Verification items for the finished model (mm, model axes). Round coordinates to 2 decimals unless told otherwise and drop trailing zeros. Order: outer loops, then holes, each group sorted by start corner. A loop starts at its lowest first (then second) coordinate and runs counter-clockwise, first axis right, second up. Notation, with made-up numbers: M 80,7.5 L 134,7.5 A17 cw 134,18.5 Z; hole C -29,6.5 d9. An arc over 180 degrees is marked long. Use one line per item in the form item = value. Start each with the question number.
Item 1: Cross-section at B-B on x = 26. Enter the section's corners in (y, z), then the cut area to 3 significant figures.
Item 2: Cross-section at A-A on y = 30. Enter the section's corners in (x, z).
Item 3: Thickness scan on probe 1 along X at (y, z) = (19, 10); probe 2 along X at (y, z) = (72.5, 7.75); probe 3 along Y at (x, z) = (2.5, 8). Record the ranges inside material, lowest first. Write a range as [from, to].
Item 4: Go/stop test with flat-tipped pins: pin 1 Ø2 at (x, y) = (-2.5, -17.5) entering from -Z; pin 2 Ø3 at (x, y) = (25.58, 30) entering from +Z. Record where each tip stops, or that it passes through.
Item 5: Cross-section at C-C on x = -23.5. Enter the section's corners in (y, z).
Item 6: Release check for a two-part mould opening along Y. For faces 1 (the cylindrical face through (2.24, -66.03, 9.86)), 2 (the cylindrical face through (-24.96, 68.06, 9.86)), 3 (the flat face through (-1, 82, 10)), 4 (the flat face through (-37.5, -1, 10)) record: +Y half, -Y half, draft (parallel to the pull), parting line (faces both ways), or undercut.
from build123d import *

# Parameters (mm, degrees)
SKETCH1_W           = 75
SKETCH1_H           = 164
SKETCH1_R           = 1.4
SKETCH1_R_2         = 2.5
BOSS_EXTRUDE1_DEPTH = 20
SKETCH2_R           = 1.4
CUT_EXTRUDE1_DEPTH  = 165


with BuildPart() as part:
    # Sketch1 → Boss-Extrude1 (new body)
    with BuildSketch(Plane.XY):
        Rectangle(SKETCH1_W, SKETCH1_H)
        with Locations((-32.5324139, -64.662730375)):
            Circle(SKETCH1_R, mode=Mode.SUBTRACT)
        with Locations((32.436706201, -64.662730375)):
            Circle(SKETCH1_R, mode=Mode.SUBTRACT)
        with Locations((2.542, -64.662730375)):
            Circle(SKETCH1_R, mode=Mode.SUBTRACT)
        with Locations((25.583768895, 30)):
            Circle(SKETCH1_R_2, mode=Mode.SUBTRACT)
        with Locations((-24.416231105, 70.5)):
            Circle(SKETCH1_R_2, mode=Mode.SUBTRACT)
        with Locations((25.583768895, 70.5)):
            Circle(SKETCH1_R_2, mode=Mode.SUBTRACT)
        with Locations((-24.416231105, 30)):
            Circle(SKETCH1_R_2, mode=Mode.SUBTRACT)
    extrude(amount=BOSS_EXTRUDE1_DEPTH)

    # Sketch2 → Cut-Extrude1 (cut, through all)
    with BuildSketch(Plane(origin=(0, 82, 0), x_dir=(1, 0, 0), z_dir=(0, 1, 0))):
        with Locations((15.509889123, -9.995038215)):
            Circle(SKETCH2_R)
        with Locations((-15.490110877, -9.995038215)):
            Circle(SKETCH2_R)
    extrude(amount=-CUT_EXTRUDE1_DEPTH, mode=Mode.SUBTRACT)


solid = part.part
Output values:
q1.outline = M -82,0 L 27.53,0 L 27.53,20 L -82,20 Z; M 32.47,0 L 68.03,0 L 68.03,20 L 32.47,20 Z; M 72.97,0 L 82,0 L 82,20 L 72.97,20 Z
q1.area = 3,080 mm2
q2.outline = M -37.5,0 L -26.92,0 L -26.92,20 L -37.5,20 Z; M -21.92,0 L 23.08,0 L 23.08,20 L -21.92,20 Z; M 28.08,0 L 37.5,0 L 37.5,20 L 28.08,20 Z; hole C -15.49,10 d2.8; hole C 15.51,10 d2.8
q3.probe_1 = [-37.5, -16.89], [-14.09, 14.11], [16.91, 37.5]
q3.probe_2 = [-37.5, -25.92], [-22.92, 24.08], [27.08, 37.5]
q3.probe_3 = [-82, -66.06], [-63.26, 82]
q4.pin_1 = 0
q4.pin_2 = through
q5.outline = M -82,0 L 27.67,0 L 27.67,20 L -82,20 Z; M 32.33,0 L 68.17,0 L 68.17,20 L 32.33,20 Z; M 72.83,0 L 82,0 L 82,20 L 72.83,20 Z
q6.face_1 = undercut
q6.face_2 = undercut
q6.face_3 = +Y half
q6.face_4 = draft
